Verification items for this drawing (mm, ordinates from the low corner). A direction names the side the tool comes from. Round coordinates to 2 decimals unless told otherwise and drop trailing zeros. Order: outer loops, then holes, each group sorted by start corner. A loop starts at its lowest first (then second) coordinate and runs counter-clockwise, first axis right, second up. Notation, with made-up numbers: (63.5, 57.5) -> (103.5, 57.5) arc R20 ccw to (103.5, 62.5) -> close; hole circle Ø8 at (25, 0.5). An arc over 180 degrees is marked (long way). Use a Markdown table: item, result. Add a question column.
Item 1: Sectioned sample at D-D, the plane z = 0.5. Record the cut outline in (x, y) (1 decimal).
Item 2: Sectioned sample at B-B, the plane y = 6.75. Record the cut outline in (x, z) (1 decimal).
Item 3: Set-up check for the marked faces 1 and 2: record each of +Z, -Z, +X, -X, +Y, -Y from which the full face is reachable in a straight line by a thin tool's end or side.
Item 4: Material ranges on probe 1 along X at (y, z) = (2, 4); probe 2 along Z at (x, y) = (4, 5.5); probe 3 along X at (y, z) = (6, 3.25) (1 decimal), recorded low to high. Write a range as [from, to].
Item 5: Mould release check, pull along X, two halves, no side actions. Record for the marked faces 3, 4, 5 and 6: pulls with the +X half, pulls with the -X half, needs draft (parallel to the pull), parting line crosses it, or undercut.
Item 6: Gauge pin test, flat end, axial feed: pin 1 Ø3 at (x, z) = (24, 4) entering from +Y. Record the tip position at first contact, or that the pin passes through.
Item 7: Sectioned sample at A-A, the plane z = 4. State how many separate pieces and enclosed holes the cut face has.
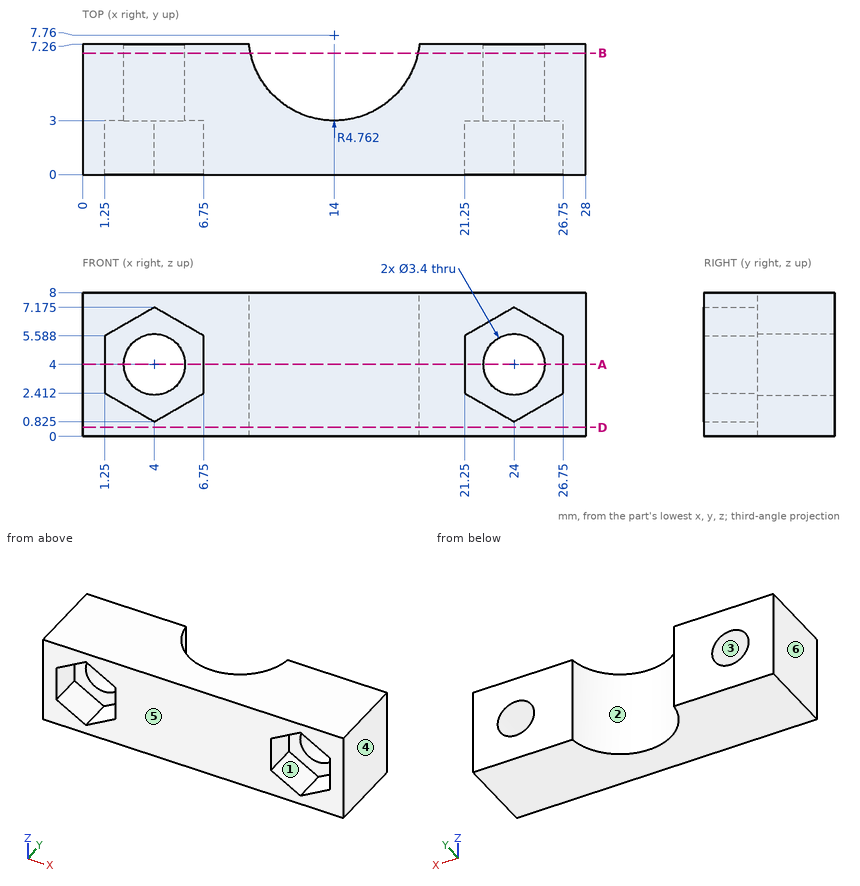
Found:
| question | item | result |
|---|---|---|
| 1 | outline | (0, 0) -> (28, 0) -> (28, 7.3) -> (18.7, 7.3) arc R4.8 cw to (9.3, 7.3) -> (0, 7.3) -> close |
| 2 | outline | (0, 0) -> (9.3, 0) -> (9.3, 8) -> (0, 8) -> close; (18.7, 0) -> (28, 0) -> (28, 8) -> (18.7, 8) -> close; hole circle Ø3.4 at (4, 4); hole circle Ø3.4 at (24, 4) |
| 3 | face 1 | -Y |
| 3 | face 2 | +Z, -Z, +Y |
| 4 | probe 1 | x = [0, 1.25], [6.75, 21.25], [26.75, 28] |
| 4 | probe 2 | z = [0, 2.3], [5.7, 8] |
| 4 | probe 3 | x = [0, 2.5], [5.5, 9.6], [18.4, 22.5], [25.5, 28] |
| 5 | face 3 | undercut |
| 5 | face 4 | pulls with the +X half |
| 5 | face 5 | needs draft |
| 5 | face 6 | pulls with the -X half |
| 6 | pin 1 | passes through |
| 7 | separate pieces | 3 |
| 7 | enclosed holes | 0 |
